from build123d import *

# Parameters (mm, degrees)
FILLET1_R              = 12.7
F_10_CLEARANCE_HOLE1_D = 5.1054


with BuildPart() as part:
    # Sketch1 → Revolve1 (revolve)
    with BuildSketch(Plane.XY, mode=Mode.PRIVATE) as revolve1_sk:
        Polygon((0, 0), (152.4, 0), (152.4, 114.3), (150.749, 114.3), (150.749, 1.5748), (0, 1.5748), align=None)
    revolve(revolve1_sk.sketch.rotate(Axis((0, 0, 0), (0, 1, 0)), 90), axis=Axis((0, 0, 0), (0, 1, 0)))

    # Fillet1
    fillet1_edges = [part.edges().sort_by_distance(p)[0] for p in [
        (0, 1.5748, 150.749),
        (0, 0, 152.4),
    ]]
    fillet(fillet1_edges, radius=FILLET1_R)

    # #10 Clearance Hole1 (through all)
    with Locations(Plane.XZ):
        with Locations((0, 38.1), (32.995567884, 19.05), (32.995567884, -19.05), (0, -38.1), (-32.995567884, -19.05), (-32.995567884, 19.05)):
            Hole(F_10_CLEARANCE_HOLE1_D / 2)


solid = part.part
Verification items for the finished model (mm, model axes). A direction names the side the tool comes from. Round coordinates to 2 decimals unless told otherwise and drop trailing zeros. Loops run counter-clockwise (first coordinate to the right, second up) from the corner with the lowest first, then second, coordinate; pieces in that order, holes last. Notation, with made-up numbers: (79.5, 15) - (96.5, 15) arc R23 ccw to (96.5, 23) - close; hole circle Ø11 at (81, 86). An arc over 180 degrees is marked (long way). Answer in a Markdown table with one row per item. Add a question column.
Q1. Material ranges on line 1 (X direction, y = 64.5, z = 1.5); line 2 (Y direction, x = -98.5, z = -63); line 3 (Z direction, x = 85, y = 72), recorded low to high.
Q2. Release check for a two-part mould opening along X. For faces 3 (the face through (-2, 1.575, 2)), 4 (the face through (-2, 0, -2)), 5 (the face through (148.776, 64.211, 33.037)) record: pulls with the +X half, pulls with the -X half, needs draft (parallel to the pull), parting line crosses it, or undercut.
Q3. Tool access check on faces 1 (the face through (-35, 114.3, 147)), 2 (the face through (-127.112, 63.587, -81.042)). Record the directions out of +Z, -Z, +X, -X, +Y, -Y that give a thin tool (end or side, any length) a straight path to the whole face; none if there is none.
Q4. Section check A-A on z = 0. Enter the section's corners in (x, y).
Q5. Section check B-B on y = 36. Enter the section's corners in (x, z), plus the area to 3 significant figures.
Q6. Gauge pin test, flat ends, axial feed: pin 1 (1.5 mm diameter, centred on x = 63.5, y = 81.5, fed in from +Z); pin 2 (6 mm diameter, centred on x = -33, z = 19.05, fed in from -Y); pin 3 (12 mm diameter, centred on y = 67, z = 113, fed in from -X); pin 4 (1 mm diameter, centred on y = 57.5, z = 117.5, fed in from -X). Record the tip position at first contact, or that the pin passes through.
Found:
| question | item | result |
|---|---|---|
| 1 | line 1 | x = -152.39 to -150.74, 150.74 to 152.39 |
| 1 | line 2 | y = 0 to 1.57 |
| 1 | line 3 | z = -126.49 to -124.5, 124.5 to 126.49 |
| 2 | face 3 | undercut |
| 2 | face 4 | needs draft |
| 2 | face 5 | parting line crosses it |
| 3 | face 1 | +Z, -Z, +X, -X, +Y |
| 3 | face 2 | +Y |
| 4 | outline | (-152.4, 12.7) arc R12.7 ccw to (-139.7, 0) - (139.7, 0) arc R12.7 ccw to (152.4, 12.7) - (152.4, 114.3) - (150.75, 114.3) - (150.75, 14.27) arc R12.7 cw to (138.05, 1.57) - (-138.05, 1.57) arc R12.7 cw to (-150.75, 14.27) - (-150.75, 114.3) - (-152.4, 114.3) - close |
| 5 | outline | circle Ø304.8 at (0, 0); hole circle Ø301.5 at (0, 0) |
| 5 | area | 1,570 mm² |
| 6 | pin 1 | stops at z = 138.88 |
| 6 | pin 2 | stops at y = 0 |
| 6 | pin 3 | stops at x = -108.52 |
| 6 | pin 4 | stops at x = -97.66 |
